Design review of the part built by this model. Coordinates are the model's own, in mm. Face numbers are marked on the shaded views. A direction names the side the tool comes from. Coordinates: 2 decimals unless noted, no trailing zeros. Loops run counter-clockwise (first coordinate to the right, second up) from the corner with the lowest first, then second, coordinate; pieces in that order, holes last.
Q1. Add section B-B on x = 1.25. Give the boundary of the cut face in (y, z), and give its area (3 significant figures).
Q2. Add section A-A on y = 0. Give the boundary of the cut face in (x, z), and give its area (3 significant figures).
Q3. Machinability: for the marked faces 1, 2 and 3, which of the approach directions +Z, -Z, +X, -X, +Y, -Y give a long, thin tool a straight path to every point of the face, cutting with its end or side? Answer none if there is none.
Q4. For P1, Ø1.5, axis at x = -1, y = 6.5, coming from the +Z side; P2, Ø1, axis at x = 0, z = -1, coming from the +Y side; P3, Ø0.6, axis at x = 1, z = 2.5, coming from the -Y side, all flat-tipped, find the tip position at first contact; note any pin that passes through.
Q5. Wall thickness on probe 1 along Z at (x, y) = (-1.1, 9); probe 2 along Z at (x, y) = (-0.7, -7); probe 3 along Y at (x, z) = (-1.55, 0.8): over which ranges is each line inside the solid? List them lowest first.
Q6. Add section D-D on z = 1.35. Give the boundary of the cut face in (x, y) (3 decimals), and give its area (3 significant figures).
Q7. Add section C-C on z = -0.7. Give the boundary of the cut face in (x, y), and give its area (3 significant figures).
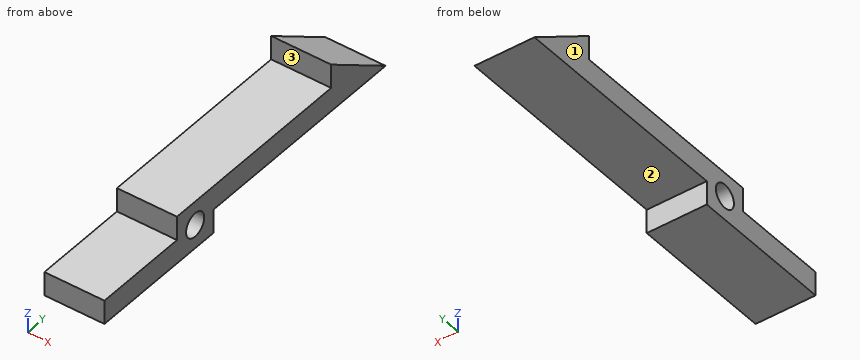
```python
from build123d import *

# Parameters (mm, degrees)
SKIZZE1_R               = 1
LINEAR_AUSTRAGEN1_DEPTH = 2.5


with BuildPart() as part:
    # Skizze1 → Linear austragen1 (new body, symmetric)
    with BuildSketch(Plane(origin=(0, 0, 0), x_dir=(0, 0, -1), z_dir=(1, 0, 0))):
        Polygon((0, 21), (-4, 15), (-2, 15), (-2, -2), (0, -2), (0, -10), (2, -10), (2, 2), (0, 2), align=None)
        Circle(SKIZZE1_R, mode=Mode.SUBTRACT)
    extrude(amount=LINEAR_AUSTRAGEN1_DEPTH, both=True)


solid = part.part
```
Entries:
1. outline: (-10, -2) - (2, -2) - (2, 0) - (21, 0) - (15, 4) - (15, 2) - (-2, 2) - (-2, 0) - (-10, 0) - close; hole circle Ø2 at (0, 0)
1. area: 66.9 mm2
2. outline: (-2.5, -2) - (2.5, -2) - (2.5, -1) - (-2.5, -1) - close; (-2.5, 1) - (2.5, 1) - (2.5, 2) - (-2.5, 2) - close
2. area: 10.0 mm2
3. face 1: +Z, -Z, -X, +Y, -Y
3. face 2: -Z, +X, -X, +Y
3. face 3: +Z, +X, -X, -Y
4. P1: stops at z = 2
4. P2: stops at y = 2
4. P3: stops at y = 15
5. probe 1: z = 0 to 2
5. probe 2: z = -2 to 0
5. probe 3: y = -2 to -0.6, 0.6 to 19.8
6. outline: (-2.5, -2) - (2.5, -2) - (2.5, 18.975) - (-2.5, 18.975) - close
6. area: 105 mm2
7. outline: (-2.5, -10) - (2.5, -10) - (2.5, -0.71) - (-2.5, -0.71) - close; (-2.5, 0.71) - (2.5, 0.71) - (2.5, 2) - (-2.5, 2) - close
7. area: 52.9 mm2
